```python
from build123d import *

# Parameters (mm, degrees)
F0_R     = 8
F1_DEPTH = 11
F2_W     = 11
F2_H     = 32
F3_DEPTH = 20
F5_R     = 9
F6_DEPTH = 32
F7_SIZE  = 1
F8_R     = 2


with BuildPart() as f1:
    # F0 (on Front) → F1 (new body)
    with BuildSketch(Plane.XZ):
        with BuildLine():
            Line((-36, 0), (-11, 0))
            Line((-11, 0), (-11, 32))
            Line((-11, 32), (-36, 32))
            ThreePointArc((-36, 32), (-52, 16), (-36, 0))
        make_face()
        with Locations((-36, 16)):
            Circle(F0_R, mode=Mode.SUBTRACT)
    extrude(amount=-F1_DEPTH)

    # F2 (on Front) → F3 (join)
    with BuildSketch(Plane.XZ):
        with Locations((-5.5, 16)):
            Rectangle(F2_W, F2_H)
    extrude(amount=-F3_DEPTH)

    # F4: F1 across face


with BuildPart() as f1_1:
    add(f1.part)
    add(f1.part.mirror(Plane(origin=(-5.5, 20, 16), x_dir=(1, 0, 0), z_dir=(0, 1, 0))))

    # F5 (on face) → F6 (join)
    with BuildSketch(Plane.YZ):
        with Locations((20, 16)):
            Circle(F5_R)
    extrude(amount=F6_DEPTH)

    # F7
    f7_edges = [f1_1.edges().sort_by_distance(p)[0] for p in [
        (-44, 0, 16),
        (-44, 11, 16),
        (-44, 29, 16),
        (-44, 40, 16),
    ]]
    chamfer(f7_edges, length=F7_SIZE)

    # F8
    f8_edges = [f1_1.edges().sort_by_distance(p)[0] for p in [
        (32, 11, 16),
        (0, 20, 32),
        (0, 40, 16),
        (0, 20, 0),
        (0, 0, 16),
        (-36, 5.5, 32),
        (-18, 0, 32),
        (-18, 40, 32),
        (-36, 34.5, 32),
        (-23.5, 29, 32),
        (-11, 20, 32),
        (-23.5, 11, 32),
    ]]
    fillet(f8_edges, radius=F8_R)


solid = f1_1.part
```
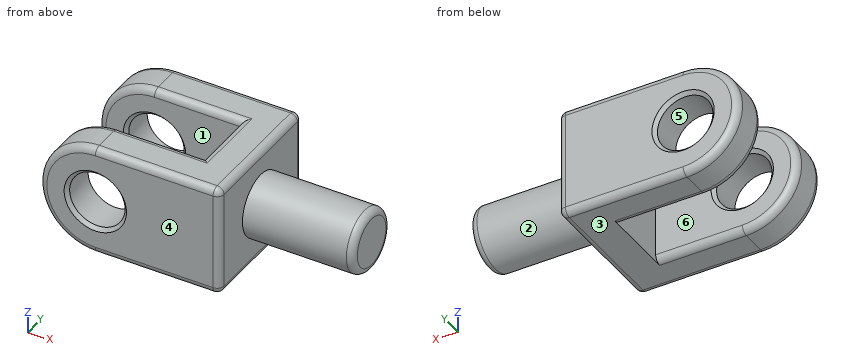
Work out the finished part from the listing and answer in its coordinate system (mm). Face numbers are marked on the shaded views. A direction names the side the tool comes from. Round coordinates to 2 decimals unless told otherwise and drop trailing zeros. Write each loop counter-clockwise with the first axis right and the second up, starting at its lowest first coordinate (ties: lowest second). Pieces come first, ordered by that corner, then holes. Notation, with made-up numbers: (24.25, 48) - (72.25, 48) arc R17 ccw to (72.25, 66) - close; hole circle Ø6 at (85.5, 2.5). An arc over 180 degrees is marked (long way). Return JSON: item names as keys, results as strings. Group by question number.
Q1. The part is cut by section B-B on z = 16. Count the separate pieces of the cut face and the enclosed holes in it, then the cut area to 3 significant figures.
Q2. Find the intervals of material crossed by L1, parallel to Z at x = -36, y = 35; L2, parallel to Y at x = -14.5, z = 17.5; L3, parallel to X at y = 17, z = 5, in increasing order.
Q3. The part is cut by section A-A on x = -13. Write down the section's boundary in (y, z).
Q4. Each of these flat-tipped pins is pushed along its axis until it touches: pin 1 Ø1 at (y, z) = (8, 26) entering from -X; pin 2 Ø4 at (y, z) = (11, 14.5) entering from -X; pin 3 Ø1 at (x, z) = (1, 4.5) entering from -Y; pin 4 Ø3 at (x, y) = (8.5, 16) entering from +Z. Where does it stop, or does it pass through?
Q5. The part is cut by section D-D on x = 14. Write down the section's boundary in (y, z), then the cut area to 3 significant figures.
Q6. For the marked faces 1, 2 and 3, determine the directions among +Z, -Z, +X, -X, +Y, -Y from which every point of the face is accessible in a straight line to the end or side of a thin tool.
Q7. The mould has two halves that part along Y. Classify the marked faces 4, 5 and 6: released by +Y, released by -Y, zero draft, split by the parting line, or undercut.
Q8. The part is cut by section C-C on y = 20. Write down the section's boundary in (x, z).
Solved:
{
 "1": {"separate pieces": "3", "enclosed holes": "0", "area": "1,560 mm²"},
 "2": {"L1": "0 to 8, 24 to 32", "L2": "0 to 11, 29 to 40", "L3": "-11 to 0"},
 "3": {"outline": "(0, 2) arc R2 ccw to (2, 0) - (9, 0) arc R2 ccw to (11, 2) - (11, 30) arc R2 ccw to (9, 32) - (2, 32) arc R2 ccw to (0, 30) - close; (29, 2) arc R2 ccw to (31, 0) - (38, 0) arc R2 ccw to (40, 2) - (40, 30) arc R2 ccw to (38, 32) - (31, 32) arc R2 ccw to (29, 30) - close"},
 "4": {"pin 1": "x = -48.87", "pin 2": "x = -51.98", "pin 3": "through", "pin 4": "z = 24.65"},
 "5": {"outline": "circle Ø18 at (20, 16)", "area": "254 mm²"},
 "6": {"face 1": "+Z, -Z, -X", "face 2": "+X", "face 3": "-Z, +X, -X, +Y, -Y"},
 "7": {"face 4": "released by -Y", "face 5": "zero draft", "face 6": "undercut"},
 "8": {"outline": "(-11, 0) - (-2, 0) arc R2 ccw to (0, 2) - (0, 7) - (30, 7) arc R2 ccw to (32, 9) - (32, 23) arc R2 ccw to (30, 25) - (0, 25) - (0, 30) arc R2 ccw to (-2, 32) - (-9, 32) arc R2 ccw to (-11, 30) - close"}
}
